from build123d import *

# Parameters (mm, degrees)
SKETCH1_W              = 15
SKETCH1_H              = 15
SKETCH1_W_2            = 12
SKETCH1_H_2            = 12
EXTRUDE_THIN1_DEPTH    = 80.79
CUT_EXTRUDE1_OUTLINE_R = 1.5
CUT_EXTRUDE1_DEPTH     = 15
SKETCH3_R              = 1.5
CUT_EXTRUDE2_DEPTH     = 84.528582533


# Read off the part's stored shape, not the designer's step: Cut-Extrude1
with BuildPart() as part:
    # Sketch1 → Extrude-Thin1 (new body)
    with BuildSketch(Plane(origin=(0, 0, 0), x_dir=(1, 0, 0), z_dir=(0, 1, 0))):
        with Locations((7.5, 7.5)):
            Rectangle(SKETCH1_W, SKETCH1_H)
        with Locations((7.5, 7.5)):
            Rectangle(SKETCH1_W_2, SKETCH1_H_2, mode=Mode.SUBTRACT)
    extrude(amount=EXTRUDE_THIN1_DEPTH)

    # Cut-Extrude1 outline → Cut-Extrude1 (cut)
    with BuildSketch(Plane.YZ):
        with Locations((73.291264227, -7.5)):
            Circle(CUT_EXTRUDE1_OUTLINE_R)
        with Locations((7.501264227, -7.5)):
            Circle(CUT_EXTRUDE1_OUTLINE_R)
    extrude(amount=CUT_EXTRUDE1_DEPTH, mode=Mode.SUBTRACT)

    # Sketch3 → Cut-Extrude2 (cut, through all)
    with BuildSketch(Plane.XY):
        with Locations((7.5, 15)):
            Circle(SKETCH3_R)
        with Locations((7.5, 65.79)):
            Circle(SKETCH3_R)
    extrude(amount=-CUT_EXTRUDE2_DEPTH, mode=Mode.SUBTRACT)


solid = part.part
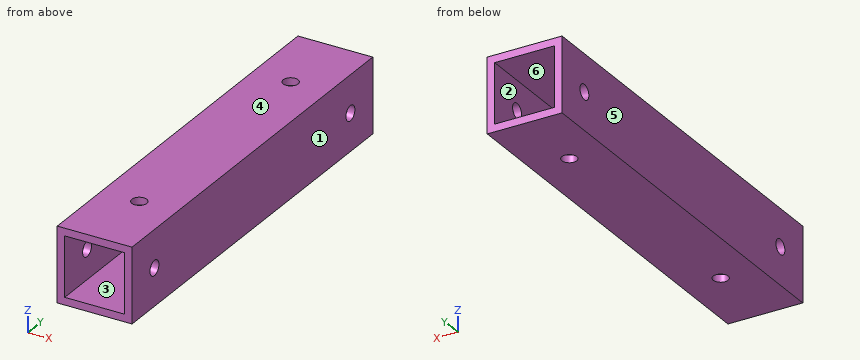
Input: part model. Units: mm. Frame: model coordinates. Face numbers are marked on the shaded views. A direction names the side the tool comes from. Give positions to 0.01 mm unless a question says otherwise; leave off trailing zeros. Order: outer loops, then holes, each group sorted by start corner. A loop starts at its lowest first (then second) coordinate and runs counter-clockwise, first axis right, second up. Notation, with made-up numbers: (24, -28) - (68, -28) arc R27 ccw to (68, 8) - close; hole circle Ø8 at (66.5, 41). An arc over 180 degrees is marked (long way). Write each question's results on one line, items separated by ' | '.
Item 1: Contact query for flat-ended pins moving along their axis: pin 1 Ø1.8 at (y, z) = (73.29, -7.5) entering from -X; pin 2 Ø3.5 at (x, y) = (7.5, 15) entering from +Z. Output: stop coordinate, or through.
A:
pin 1: passes through | pin 2: stops at z = 0
Item 2: Section A-A (x = 4). Return loops of the section in (y, z).
A:
outline: (0, -15) - (80.79, -15) - (80.79, -13.5) - (0, -13.5) - close; (0, -1.5) - (80.79, -1.5) - (80.79, 0) - (0, 0) - close
Item 3: Section D-D (y = 65.79). Return loops of the section in (x, z).
A:
outline: (0, -15) - (6, -15) - (6, -13.5) - (1.5, -13.5) - (1.5, -1.5) - (6, -1.5) - (6, 0) - (0, 0) - close; (9, -15) - (15, -15) - (15, 0) - (9, 0) - (9, -1.5) - (13.5, -1.5) - (13.5, -13.5) - (9, -13.5) - close
Item 4: Material intervals for line 1 along Y through (x, z) = (7.5, -1.15); line 2 along Y through (x, z) = (14.2, -7.5); line 3 along Z through (x, y) = (6.75, 8.5), sorted ascending.
A:
line 1: y = 0 to 13.5, 16.5 to 64.29, 67.29 to 80.79 | line 2: y = 0 to 6, 9 to 71.79, 74.79 to 80.79 | line 3: z = -15 to -13.5, -1.5 to 0
Item 5: Section B-B (y = 57.5). Return loops of the section in (x, z).
A:
outline: (0, -15) - (15, -15) - (15, 0) - (0, 0) - close; hole (1.5, -13.5) - (13.5, -13.5) - (13.5, -1.5) - (1.5, -1.5) - close
Item 6: Access query for the marked faces 5 and 6. Directions: +Z, -Z, +X, -X, +Y, -Y. A direction counts if a zero-diameter tool reaches every point of the face in a straight line with its end or side. Return the directions, or none.
A:
face 5: +Z, -Z, -X, +Y, -Y | face 6: +Y, -Y
Item 7: Draft query along Z for the marked faces 1, 2, 3 and 4. Return one class per face: released by +Z, released by -Z, zero draft, split by the parting line, or undercut.
A:
face 1: zero draft | face 2: undercut | face 3: undercut | face 4: released by +Z
Item 8: Section C-C (z = -4.75). Return loops of the section in (x, y).
A:
outline: (0, 0) - (1.5, 0) - (1.5, 80.79) - (0, 80.79) - close; (13.5, 0) - (15, 0) - (15, 80.79) - (13.5, 80.79) - close
